Part model, mm, in its own coordinate system. Coordinates: 2 decimals unless noted, no trailing zeros. Loops run counter-clockwise (first coordinate to the right, second up) from the corner with the lowest first, then second, coordinate; pieces in that order, holes last. Notation, with made-up numbers: (-40, -4.75) - (-30, -4.75) arc R33 ccw to (-30, 28.25) - close; hole circle Ø2 at (16, -17). An arc over 180 degrees is marked (long way). Use a Markdown table: item, result. Add a question column.
1) Probe probe 1 along Z at (x, y) = (68, 2.15); probe 2 along Z at (x, y) = (0, 0.8); probe 3 along Z at (x, y) = (42.5, 1.6). List the from-to ranges inside material, lowest first. Write a range as [from, to].
2) Band-saw the part on A-A (x = 0). Give the cut face in (y, z), plus the area to 3 significant figures.
3) Band-saw the part on C-C (z = 0). Give the cut face in (x, y).
4) Band-saw the part on B-B (y = 1.15). Give the cut face in (x, z), plus the area to 3 significant figures.
5) Band-saw the part on D-D (z = 13.5). Give the cut face in (x, y).
6) Drop a flat-ended pin along its axis: P1, Ø2.5, axis at x = 53, z = 0, coming from the +Y side. Give the stop position or say it passes through.
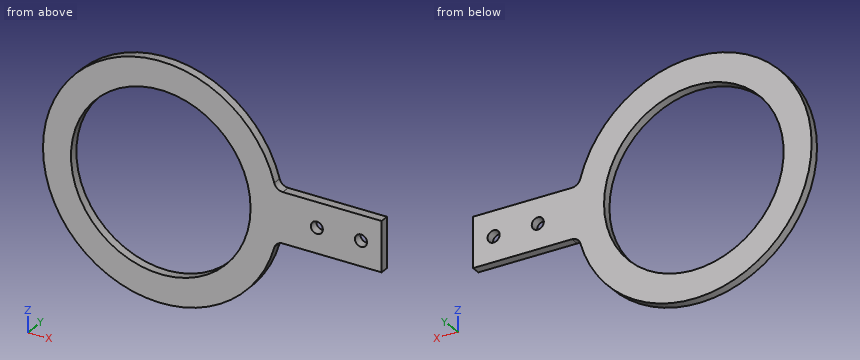
from build123d import *

# Parameters (mm, degrees)
SKETCH1_R           = 40
SKETCH1_R_2         = 30.5
BOSS_EXTRUDE1_DEPTH = 3
SKETCH2_W           = 40
SKETCH2_H           = 17
BOSS_EXTRUDE2_DEPTH = 3
SKETCH3_R           = 2.05
CUT_EXTRUDE1_DEPTH  = 4
FILLET1_R           = 3


with BuildPart() as part:
    # Sketch1 → Boss-Extrude1 (new body)
    with BuildSketch(Plane(origin=(0, 0, 0), x_dir=(1, 0, 0), z_dir=(0, 1, 0))):
        Circle(SKETCH1_R)
        Circle(SKETCH1_R_2, mode=Mode.SUBTRACT)
    extrude(amount=BOSS_EXTRUDE1_DEPTH)

    # Sketch2 → Boss-Extrude2 (add)
    with BuildSketch(Plane(origin=(0, 3, 0), x_dir=(1, 0, 0), z_dir=(0, 1, 0))):
        with Locations((55, 0)):
            Rectangle(SKETCH2_W, SKETCH2_H)
    extrude(amount=-BOSS_EXTRUDE2_DEPTH)

    # Sketch3 → Cut-Extrude1 (cut, through all)
    with BuildSketch(Plane(origin=(0, 3, 0), x_dir=(1, 0, 0), z_dir=(0, 1, 0))):
        with Locations((53, 0)):
            Circle(SKETCH3_R)
        with Locations((68, 0)):
            Circle(SKETCH3_R)
    extrude(amount=-CUT_EXTRUDE1_DEPTH, mode=Mode.SUBTRACT)

    # Fillet1
    fillet1_edges = [part.edges().sort_by_distance(p)[0] for p in [
        (39.086442662, 1.5, 8.5),
        (39.086442662, 1.5, -8.5),
    ]]
    fillet(fillet1_edges, radius=FILLET1_R)


solid = part.part
Answer block:
| question | item | result |
|---|---|---|
| 1 | probe 1 | [-8.5, -2.05], [2.05, 8.5] |
| 1 | probe 2 | [-40, -30.5], [30.5, 40] |
| 1 | probe 3 | [-8.5, 8.5] |
| 2 | outline | (0, -40) - (3, -40) - (3, -30.5) - (0, -30.5) - close; (0, 30.5) - (3, 30.5) - (3, 40) - (0, 40) - close |
| 2 | area | 57.0 mm2 |
| 3 | outline | (-40, 0) - (-30.5, 0) - (-30.5, 3) - (-40, 3) - close; (30.5, 0) - (50.95, 0) - (50.95, 3) - (30.5, 3) - close; (55.05, 0) - (65.95, 0) - (65.95, 3) - (55.05, 3) - close; (70.05, 0) - (75, 0) - (75, 3) - (70.05, 3) - close |
| 4 | outline | (38.54, -10.7) arc R3 cw to (41.43, -8.5) - (75, -8.5) - (75, 8.5) - (41.43, 8.5) arc R3 cw to (38.54, 10.7) arc R40 ccw (long way) to start; hole circle Ø61 at (0, 0); hole circle Ø4.1 at (53, 0); hole circle Ø4.1 at (68, 0) |
| 4 | area | 2,680 mm2 |
| 5 | outline | (-37.65, 0) - (-27.35, 0) - (-27.35, 3) - (-37.65, 3) - close; (27.35, 0) - (37.65, 0) - (37.65, 3) - (27.35, 3) - close |
| 6 | P1 | through |
